```python
from build123d import *

# Parameters (mm, degrees)
SKETCH1_R           = 76.2
SKETCH1_R_2         = 9.525
BOSS_EXTRUDE1_DEPTH = 25.4
SKETCH2_R           = 31.75
BOSS_EXTRUDE2_DEPTH = 22.225


with BuildPart() as part:
    # Sketch1 → Boss-Extrude1 (new body)
    with BuildSketch(Plane.XY):
        Circle(SKETCH1_R)
        Circle(SKETCH1_R_2, mode=Mode.SUBTRACT)
    extrude(amount=BOSS_EXTRUDE1_DEPTH)

    # Sketch2 → Boss-Extrude2 (add)
    with BuildSketch(Plane.XY):
        Circle(SKETCH2_R)
    extrude(amount=-BOSS_EXTRUDE2_DEPTH)


solid = part.part
```
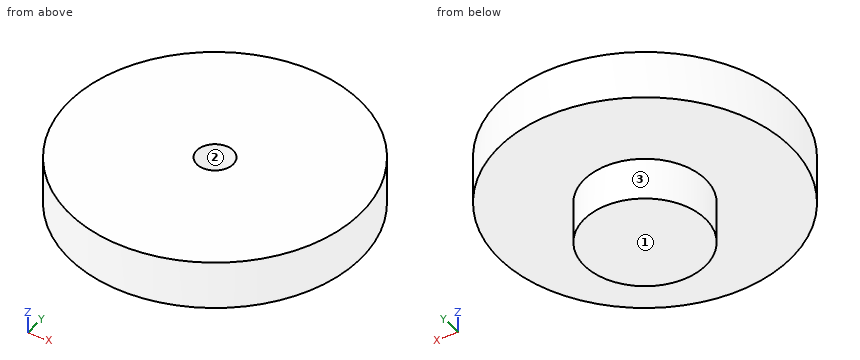
The model under review builds one solid part; all positions refer to its coordinate system, in mm. Face numbers are marked on the shaded views. A direction names the side the tool comes from. Round coordinates to 2 decimals unless told otherwise and drop trailing zeros. Order: outer loops, then holes, each group sorted by start corner. A loop starts at its lowest first (then second) coordinate and runs counter-clockwise, first axis right, second up. Notation, with made-up numbers: (-17.5, -31) - (38.5, -31) arc R13 ccw to (38.5, -22) - close; hole circle Ø3 at (34.5, 65). An arc over 180 degrees is marked (long way). Answer in a Markdown table with one row per item.
(1) Clearance check with flat-ended pins moving along their axes: P1, Ø3, axis at y = 57, z = 19, coming from the +X side; P2, Ø8, axis at y = 23.5, z = 14.5, coming from the +X side; P3, Ø9.5, axis at x = 0, y = 2.5, coming from the +Z side. State where each tip first meets the part, or that it passes through.
Result set:
| item | result |
|---|---|
| P1 | stops at x = 52.21 |
| P2 | stops at x = 73.66 |
| P3 | stops at z = 0 |
(2) Take a section at C-C on z = 17.5. Write out the cut boundary in (x, y) (3 decimals), plus the area to 3 significant figures.
Result set:
| item | result |
|---|---|
| outline | circle Ø152.4 at (0, 0); hole circle Ø19.05 at (0, 0) |
| area | 18,000 mm2 |
(3) Machinability: for the marked faces 1, 2 and 3, which of the approach directions +Z, -Z, +X, -X, +Y, -Y give a long, thin tool a straight path to every point of the face, cutting with its end or side? Answer none if there is none.
Result set:
| item | result |
|---|---|
| face 1 | -Z, +X, -X, +Y, -Y |
| face 2 | +Z |
| face 3 | -Z |
(4) Take a section at A-A on y = 0. Write out the cut boundary in (x, z) (3 decimals), plus the area to 3 significant figures.
Result set:
| item | result |
|---|---|
| outline | (-76.2, 0) - (-31.75, 0) - (-31.75, -22.225) - (31.75, -22.225) - (31.75, 0) - (76.2, 0) - (76.2, 25.4) - (9.525, 25.4) - (9.525, 0) - (-9.525, 0) - (-9.525, 25.4) - (-76.2, 25.4) - close |
| area | 4,800 mm2 |
(5) Take a section at D-D on z = -8. Write out the cut boundary in (x, y).
Result set:
| item | result |
|---|---|
| outline | circle Ø63.5 at (0, 0) |
(6) For line 1 (Y direction, x = 0, z = 11) (3 decimals); line 2 (Z direction, x = -35, y = -53); line 3 (X direction, y = 6, z = 18), list the stretches that pass through material, from the lowest coordinate up. Write a range as from..to.
Result set:
| item | result |
|---|---|
| line 1 | y = -76.2..-9.525, 9.525..76.2 |
| line 2 | z = 0..25.4 |
| line 3 | x = -75.96..-7.4, 7.4..75.96 |
